For this review, take the finished solid that the model builds, in its own axes (mm). Coordinates: 2 decimals unless noted, no trailing zeros.
```python
from build123d import *

# Parameters (mm, degrees)
BOSS_EXTRU_1_DEPTH      = 3
BOSS_EXTRU_1_DEPTH_BACK = 3
ESQUISSE1_R             = 1.5


with BuildPart() as part:
    # Esquisse1 → Boss.-Extru.1 (new, two sides: drawn at the far end of the back side and taken through both)
    with BuildSketch(Plane.XY.offset(-BOSS_EXTRU_1_DEPTH_BACK)):
        with BuildLine():
            ThreePointArc((0, 3), (-3, 0), (0, -3))
            add(Edge.make_bspline(
                [(0, -3), (34.547376403, -3), (36.359532073, 7.334799912), (43, 40)],
                knots=[0, 0, 0, 0, 1, 1, 1, 1], degree=3))
            ThreePointArc((43, 40), (40, 43), (37, 40))
            add(Edge.make_bspline(
                [(0, 3), (33.333333333, 3), (31.664729171, 12.359061598), (37, 40)],
                knots=[0, 0, 0, 0, 1, 1, 1, 1], degree=3))
        make_face()
        Circle(ESQUISSE1_R, mode=Mode.SUBTRACT)
        with Locations((40, 40)):
            Circle(ESQUISSE1_R, mode=Mode.SUBTRACT)
    extrude(amount=BOSS_EXTRU_1_DEPTH + BOSS_EXTRU_1_DEPTH_BACK)


solid = part.part
```
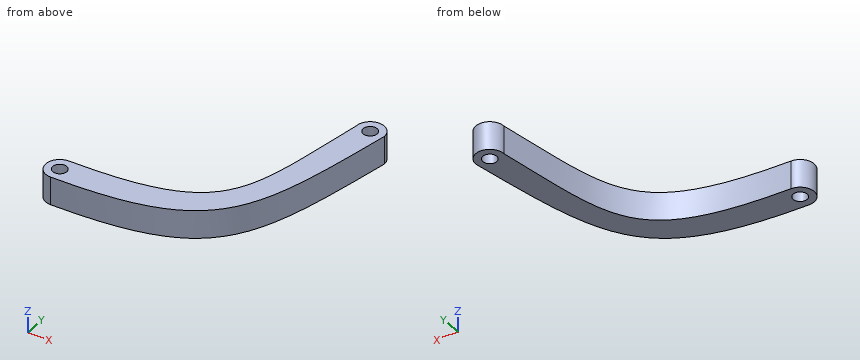
Q1. Add section A-A (z = -0.25). Give the number of separate pieces and of enclosed holes in the cut face, then the cut area to 3 significant figures.
Ans:
separate pieces: 1
enclosed holes: 2
area: 387 mm2
Q2. For probe 1 along X at (y, z) = (39, 1.25); probe 2 along X at (y, z) = (9.5, -1.75); probe 3 along Y at (x, z) = (20.5, 1), list the stretches that pass through material, from the lowest coordinate up.
Ans:
probe 1: x = 36.81 to 38.88, 41.12 to 42.8
probe 2: x = 27.57 to 34.25
probe 3: y = -0.83 to 5.33
Q3. Clearance check with flat-ended pins moving along their axes: pin 1 Ø2.5 at (x, y) = (0, 0) entering from +Z; pin 2 Ø3.5 at (x, y) = (40, 40) entering from -Z; pin 3 Ø2 at (x, z) = (14.5, -1.5) entering from -Y; pin 4 Ø2 at (x, z) = (20, 1.5) entering from -Y. State where each tip first meets the part, or that it passes through.
Ans:
pin 1: passes through
pin 2: stops at z = -3
pin 3: stops at y = -2.26
pin 4: stops at y = -1.24
